Source: CAD feature listing. Evaluate the final solid. Frame: model axes, mm. A direction names the side the tool comes from. Round coordinates to 2 decimals unless told otherwise and drop trailing zeros. Order: outer loops, then holes, each group sorted by start corner. A loop starts at its lowest first (then second) coordinate and runs counter-clockwise, first axis right, second up. Notation, with made-up numbers: (7.25, 20.5) -> (63.25, 20.5) arc R22 cw to (63.25, 55.5) -> close; hole circle Ø9 at (-37, -4). An arc over 180 degrees is marked (long way). Answer as CSV lines item,"result".
from build123d import *

# Parameters (mm, degrees)
BOSS_EXTRUDE1_DEPTH = 30
SKETCH2_R           = 1.6
CUT_EXTRUDE1_DEPTH  = 10
SKETCH3_R           = 1.6
CUT_EXTRUDE2_DEPTH  = 4


with BuildPart() as part:
    # Sketch1 → Boss-Extrude1 (new body)
    with BuildSketch(Plane.XY):
        Polygon((0, 20), (0, 0), (20, 0), (20, 2), (2, 2), (2, 20), align=None)
    extrude(amount=BOSS_EXTRUDE1_DEPTH)

    # Sketch2 → Cut-Extrude1 (cut)
    with BuildSketch(Plane(origin=(0, 0, 0), x_dir=(0, 0, -1), z_dir=(1, 0, 0))):
        with Locations((-22.5, 9.5)):
            Circle(SKETCH2_R)
        with Locations((-7.5, 9.5)):
            Circle(SKETCH2_R)
    extrude(amount=CUT_EXTRUDE1_DEPTH, mode=Mode.SUBTRACT)

    # Sketch3 → Cut-Extrude2 (cut)
    with BuildSketch(Plane(origin=(0, 0, 0), x_dir=(1, 0, 0), z_dir=(0, 1, 0))):
        with Locations((13, -10)):
            Circle(SKETCH3_R)
        with Locations((13, -20)):
            Circle(SKETCH3_R)
    extrude(amount=CUT_EXTRUDE2_DEPTH, mode=Mode.SUBTRACT)


solid = part.part
1. Section query D-D on z = 26.25. Return loops of the section in (x, y), and give its area (3 significant figures).
Results below:
outline,"(0, 0) -> (20, 0) -> (20, 2) -> (2, 2) -> (2, 20) -> (0, 20) -> close"
area,"76.0 mm2"
2. Section query A-A on y = 9.5. Return loops of the section in (x, z), and give its area (3 significant figures).
Results below:
outline,"(0, 0) -> (2, 0) -> (2, 5.9) -> (0, 5.9) -> close; (0, 9.1) -> (2, 9.1) -> (2, 20.9) -> (0, 20.9) -> close; (0, 24.1) -> (2, 24.1) -> (2, 30) -> (0, 30) -> close"
area,"47.2 mm2"
3. Pin query (flat end, axial travel): pin 1 (2 mm diameter, centred on x = 4.5, z = 25.5, fed in from -Y); pin 2 (2 mm diameter, centred on x = 17, z = 17.5, fed in from +Y); pin 3 (5.5 mm diameter, centred on y = 14.5, z = 20, fed in from +X). Return the tip coordinate at first contact, or that it passes through.
Results below:
pin 1,"y = 0"
pin 2,"y = 2"
pin 3,"x = 2"
4. Line query: L1, parallel to Z at x = 1.65, y = 9.5; L2, parallel to Z at x = 13, y = 1.15; L3, parallel to Y at x = 0.5, z = 7.5. Output: solid intervals per line, ascending. Write a range as [from, to].
Results below:
L1,"[0, 5.9], [9.1, 20.9], [24.1, 30]"
L2,"[0, 8.4], [11.6, 18.4], [21.6, 30]"
L3,"[0, 7.9], [11.1, 20]"
5. Section query B-B on z = 20. Return loops of the section in (x, y).
Results below:
outline,"(0, 0) -> (11.4, 0) -> (11.4, 2) -> (2, 2) -> (2, 20) -> (0, 20) -> close; (14.6, 0) -> (20, 0) -> (20, 2) -> (14.6, 2) -> close"
6. Section query C-C on x = 13. Return loops of the section in (y, z), and give its area (3 significant figures).
Results below:
outline,"(0, 0) -> (2, 0) -> (2, 8.4) -> (0, 8.4) -> close; (0, 11.6) -> (2, 11.6) -> (2, 18.4) -> (0, 18.4) -> close; (0, 21.6) -> (2, 21.6) -> (2, 30) -> (0, 30) -> close"
area,"47.2 mm2"
7. Reachability of faces 1 (the flat face through (11, 2, 15)), 2 (the flat face through (10, 0, 15)) from +Z, -Z, +X, -X, +Y, -Y: full face, straight path, thin tool, end or side. Return the list, or none.
Results below:
face 1,"+Z, -Z, +X, +Y"
face 2,"+Z, -Z, +X, -X, -Y"
8. Mould query, pull axis Z, two halves, no side actions, for faces 3 (the flat face through (1.8, 5.6, 30)), 4 (the flat face through (0, 10, 15)), 5 (the cylindrical face through (0.99, 7.94, 7.85)). Classes: released by +Z, released by -Z, zero draft, split by the parting line, or undercut.
Results below:
face 3,"released by +Z"
face 4,"zero draft"
face 5,"undercut"
